from build123d import *

# Parameters (mm, degrees)
BOSS_EXTRUDE1_DEPTH = 96
CUT_EXTRUDE1_DEPTH  = 101.079968026


with BuildPart() as part:
    # Sketch1 → Boss-Extrude1 (new body)
    with BuildSketch(Plane(origin=(0, 0, 0), x_dir=(0, 0, -1), z_dir=(1, 0, 0))):
        Polygon((0, 20), (0, 0), (20, 0), (20, 2), (2, 2), (2, 20), align=None)
    extrude(amount=BOSS_EXTRUDE1_DEPTH)

    # Sketch2 → Cut-Extrude1 (cut, through all)
    with BuildSketch(Plane.XY):
        Polygon((0, 0), (4.251131233, 20), (0, 20), align=None)
    extrude(amount=-CUT_EXTRUDE1_DEPTH, mode=Mode.SUBTRACT)


solid = part.part
Here's how the part is built. I have some questions about the finished solid (model axes, mm). A direction names the side the tool comes from. Round coordinates to 2 decimals unless told otherwise and drop trailing zeros. Write each loop counter-clockwise with the first axis right and the second up, starting at its lowest first coordinate (ties: lowest second). Pieces come first, ordered by that corner, then holes.
1. For faces 1 (the flat face through (47, 10, 0)), 2 (the flat face through (48, 11, -2)), which set-ups out of +Z, -Z, +X, -X, +Y, -Y let a thin tool reach every point of the face, with its end or its side?
2. Suppose I cut it at B-B (z = -6). List the corners of the cut face in (x, y) for me, and give its area (3 significant figures).
3. I need wall thicknesses on L1, parallel to Z at x = 18, y = 6.75; L2, parallel to Y at x = 22, z = -4.75. Which ranges of each line are inside material? Lowest first, please.
4. Will these pins go through, and if not, where does the flat tip stop? pin 1 Ø6 at (x, z) = (86, -17) entering from +Y; pin 2 Ø1.5 at (x, z) = (48.5, -8) entering from -Y; pin 3 Ø10 at (y, z) = (15.5, -4) entering from -X; pin 4 Ø1.5 at (y, z) = (13.5, -3) entering from -X.
5. Suppose I cut it at C-C (y = 11). List the corners of the cut face in (x, z) for me.
6. Suppose I cut it at A-A (x = 86.5). List the corners of the cut face in (y, z) for me.
Answer sheet:
1. face 1: +Z, +X, -X, +Y, -Y
1. face 2: -Z, +X, -X, +Y
2. outline: (0, 0) - (96, 0) - (96, 2) - (0.43, 2) - close
2. area: 192 mm2
3. L1: z = -2 to 0
3. L2: y = 0 to 2
4. pin 1: stops at y = 2
4. pin 2: stops at y = 0
4. pin 3: stops at x = 2.32
4. pin 4: passes through
5. outline: (2.34, -2) - (96, -2) - (96, 0) - (2.34, 0) - close
6. outline: (0, -20) - (2, -20) - (2, -2) - (20, -2) - (20, 0) - (0, 0) - close
